Part model, mm, in its own coordinate system. A direction names the side the tool comes from. Give positions to 0.01 mm unless a question says otherwise; leave off trailing zeros. Order: outer loops, then holes, each group sorted by start corner. A loop starts at its lowest first (then second) coordinate and runs counter-clockwise, first axis right, second up. Notation, with made-up numbers: (5, -20) -> (40, -20) arc R25 ccw to (40, 13) -> close; hole circle Ø6 at (24.5, 42.25). An arc over 180 degrees is marked (long way). Write item = value, one per line. Start each with the question number.
(1) Saw through at B-B, the plane x = -22. List the corners of the cut face in (y, z), then the cut area to 3 significant figures.
(2) Flat gauge pins, fed straight in: pin 1 (1.3 mm diameter, centred on x = -43.5, z = 29, fed in from -Y); pin 2 (1 mm diameter, centred on x = -1, z = -31, fed in from -Y); pin 3 (1.8 mm diameter, centred on x = -45.83, z = -30.48, fed in from +Y); pin 4 (1.6 mm diameter, centred on y = 2, z = 3, fed in from +X). Where does each tip first touch, or does it go through?
(3) Two-plate mould, pull along X, no slides. Class faces 4 (the flat face through (1, -2, -29.813)), 5 (the flat face through (-41.632, 2, -31)), 6 (the cylindrical face through (43.43, -0.161, -28.686)), 7 (the flat face through (42.77, -1, 0)): pulls with the +X half, pulls with the -X half, needs draft (parallel to the pull), parting line crosses it, or undercut.
(4) Saw through at A-A, the plane z = -6. List the corners of the cut face in (x, y).
(5) Which spindle directions (+Z, -Z, +X, -X, +Y, -Y) get a long thin tool onto all of the face, cutting with end or side? Do faces 1 (the cylindrical face through (-43.454, -0.161, -28.654)), 2 (the cylindrical face through (45.09, 0.49, -26.23)), 3 (the cylindrical face through (-43.473, -2.058, 28.63)). Say none if no direction does.
(6) Probe line 1 along X through (y, z) = (-0.45, 21.5); line 2 along Z through (x, y) = (-11.5, -0.15); line 3 along X through (y, z) = (-2.2, -30.48). List the from-to ranges inside material, lowest first. Write a range as from..to.
from build123d import *

# Parameters (mm, degrees)
SKETCH1_W             = 83.263532188
SKETCH1_H             = 2
BOSS_EXTRUDE1_DEPTH   = 2.4732
BOSS_EXTRUDE1_2_DEPTH = 2.4732
SKETCH1_3_W           = 85.5392
SKETCH1_3_H           = 56.126
BOSS_EXTRUDE2_DEPTH   = 1
BOSS_EXTRUDE3_START   = -3.29023885
SKETCH1_4_W           = 85.5392
SKETCH1_4_H           = 56.126
BOSS_EXTRUDE3_DEPTH   = 3.29023885
BOSS_EXTRUDE4_START   = -3.290239
BOSS_EXTRUDE4_DEPTH   = 2
FILLET1_R             = 2
FILLET2_R             = 2
SKETCH2_R             = 3
CUT_EXTRUDE1_DEPTH    = 3
CUT_EXTRUDE2_START    = -2
SKETCH2_3_R           = 3
CUT_EXTRUDE2_DEPTH    = 2.5


with BuildPart() as part:
    # Sketch1 → Boss-Extrude1 (new body)
    with BuildSketch(Plane(origin=(0, 0, 0), x_dir=(1, 0, 0), z_dir=(0, 1, 0))):
        with Locations((0, 30.813)):
            Rectangle(SKETCH1_W, SKETCH1_H)
    extrude(amount=BOSS_EXTRUDE1_DEPTH)



with BuildPart() as body_2:
    # Sketch1 → Boss-Extrude1 2 (new body)
    with BuildSketch(Plane(origin=(0, 0, 0), x_dir=(1, 0, 0), z_dir=(0, 1, 0))):
        Polygon((-44.5196, -29.813), (-44.5196, 25.629766094), (-46.5196, 25.629766094), (-46.5196, -31.813), (46.5196, -31.813), (46.5196, 25.629766094), (44.5196, 25.629766094), (44.5196, -29.813), align=None)
    extrude(amount=BOSS_EXTRUDE1_2_DEPTH)


with BuildPart() as part_1:
    add(part.part)

    add(body_2.part)  # Boss-Extrude2 merges body 2
    # Sketch1<3> → Boss-Extrude2 (add)
    with BuildSketch(Plane(origin=(0, 0, 0), x_dir=(1, 0, 0), z_dir=(0, 1, 0))):
        with BuildLine():
            Line((41.631766094, 29.813), (-41.631766094, 29.813))
            Line((-41.631766094, 29.813), (-43.424920204, 29.813))
            ThreePointArc((-43.424920204, 29.813), (-43.834386894, 28.979884149), (-44.5196, 28.353603069))
            Line((-44.5196, 28.353603069), (-44.5196, 25.629766094))
            Line((-44.5196, 25.629766094), (-44.5196, -29.813))
            Line((-44.5196, -29.813), (44.5196, -29.813))
            Line((44.5196, -29.813), (44.5196, 25.629766094))
            Line((44.5196, 25.629766094), (44.5196, 28.353603069))
            ThreePointArc((44.5196, 28.353603069), (43.834386894, 28.979884149), (43.424920204, 29.813))
            Line((43.424920204, 29.813), (41.631766094, 29.813))
        make_face()
        Rectangle(SKETCH1_3_W, SKETCH1_3_H, mode=Mode.SUBTRACT)
    extrude(amount=BOSS_EXTRUDE2_DEPTH)

    # Sketch1<4> → Boss-Extrude3 (add)
    with BuildSketch(Plane(origin=(0, 0, 0), x_dir=(1, 0, 0), z_dir=(0, 1, 0)).offset(BOSS_EXTRUDE3_START)):
        with BuildLine():
            Line((41.631766094, 29.813), (-41.631766094, 29.813))
            Line((-41.631766094, 29.813), (-43.424920204, 29.813))
            ThreePointArc((-43.424920204, 29.813), (-43.834386894, 28.979884149), (-44.5196, 28.353603069))
            Line((-44.5196, 28.353603069), (-44.5196, 25.629766094))
            Line((-44.5196, 25.629766094), (-44.5196, -29.813))
            Line((-44.5196, -29.813), (44.5196, -29.813))
            Line((44.5196, -29.813), (44.5196, 25.629766094))
            Line((44.5196, 25.629766094), (44.5196, 28.353603069))
            ThreePointArc((44.5196, 28.353603069), (43.834386894, 28.979884149), (43.424920204, 29.813))
            Line((43.424920204, 29.813), (41.631766094, 29.813))
        make_face()
        Rectangle(SKETCH1_4_W, SKETCH1_4_H, mode=Mode.SUBTRACT)
    extrude(amount=BOSS_EXTRUDE3_DEPTH)

    # Sketch1<5> → Boss-Extrude4 (add)
    with BuildSketch(Plane(origin=(0, 0, 0), x_dir=(1, 0, 0), z_dir=(0, 1, 0)).offset(BOSS_EXTRUDE4_START)):
        with BuildLine():
            ThreePointArc((-43.3343, 30.48), (-43.524601169, 31.436708581), (-44.066533047, 32.247766953))
            ThreePointArc((-44.066533047, 32.247766953), (-47.602066953, 32.247766953), (-47.602066953, 28.712233047))
            ThreePointArc((-47.602066953, 28.712233047), (-46.123213969, 27.996750371), (-44.5196, 28.353603069))
            Line((-44.5196, 28.353603069), (-44.5196, 29.757806183))
            ThreePointArc((-44.5196, 29.757806183), (-47.287236681, 30.852793509), (-44.3343, 30.48))
            ThreePointArc((-44.3343, 30.48), (-44.373937666, 30.137448026), (-44.490755806, 29.813))
            Line((-44.490755806, 29.813), (-43.424920204, 29.813))
            ThreePointArc((-43.424920204, 29.813), (-43.357058642, 30.143436105), (-43.3343, 30.48))
        make_face()
        with BuildLine():
            ThreePointArc((-44.5196, 28.353603069), (-43.834386894, 28.979884149), (-43.424920204, 29.813))
            Line((-43.424920204, 29.813), (-44.490755806, 29.813))
            ThreePointArc((-44.490755806, 29.813), (-44.504891433, 29.785253383), (-44.5196, 29.757806183))
            Line((-44.5196, 29.757806183), (-44.5196, 28.353603069))
        make_face()
        with BuildLine():
            ThreePointArc((-44.5196, 28.353603069), (-46.123213969, 27.996750371), (-47.602066953, 28.712233047))
            Line((-47.602066953, 28.712233047), (-44.5196, 25.629766094))
            Line((-44.5196, 25.629766094), (-44.5196, 28.353603069))
        make_face()
        with BuildLine():
            Line((-41.631766094, 29.813), (-44.066533047, 32.247766953))
            ThreePointArc((-44.066533047, 32.247766953), (-43.524601169, 31.436708581), (-43.3343, 30.48))
            ThreePointArc((-43.3343, 30.48), (-43.357058642, 30.143436105), (-43.424920204, 29.813))
            Line((-43.424920204, 29.813), (-41.631766094, 29.813))
        make_face()
        with BuildLine():
            ThreePointArc((44.066533047, 32.247766953), (43.416829986, 31.117054732), (43.424920204, 29.813))
            Line((43.424920204, 29.813), (44.490755806, 29.813))
            ThreePointArc((44.490755806, 29.813), (45.491748026, 31.940362334), (47.3343, 30.48))
            ThreePointArc((47.3343, 30.48), (46.207093509, 29.027063319), (44.5196, 29.757806183))
            Line((44.5196, 29.757806183), (44.5196, 28.353603069))
            ThreePointArc((44.5196, 28.353603069), (46.123213969, 27.996750371), (47.602066953, 28.712233047))
            ThreePointArc((47.602066953, 28.712233047), (48.143998831, 29.523291419), (48.3343, 30.48))
            ThreePointArc((48.3343, 30.48), (46.791008581, 32.789698831), (44.066533047, 32.247766953))
        make_face()
        with BuildLine():
            Line((44.490755806, 29.813), (43.424920204, 29.813))
            ThreePointArc((43.424920204, 29.813), (43.834386894, 28.979884149), (44.5196, 28.353603069))
            Line((44.5196, 28.353603069), (44.5196, 29.757806183))
            ThreePointArc((44.5196, 29.757806183), (44.504891433, 29.785253383), (44.490755806, 29.813))
        make_face()
        with BuildLine():
            Line((44.066533047, 32.247766953), (41.631766094, 29.813))
            Line((41.631766094, 29.813), (43.424920204, 29.813))
            ThreePointArc((43.424920204, 29.813), (43.416829986, 31.117054732), (44.066533047, 32.247766953))
        make_face()
        with BuildLine():
            ThreePointArc((47.602066953, 28.712233047), (46.123213969, 27.996750371), (44.5196, 28.353603069))
            Line((44.5196, 28.353603069), (44.5196, 25.629766094))
            Line((44.5196, 25.629766094), (47.602066953, 28.712233047))
        make_face()
    extrude(amount=BOSS_EXTRUDE4_DEPTH)

    # Fillet1
    # the kernel refuses this fillet: 2 mm, written as the material it adds along each edge
    with BuildSketch(Plane(origin=(44.5196, 0, -25.629766094), x_dir=(0, 0, -1), z_dir=(0, 1, 0))) as fillet1_piece_1:
        with BuildLine():
            CenterArc((FILLET1_R, -FILLET1_R), FILLET1_R, 90, 90)
            Line((0, -FILLET1_R), (0, 0))
            Line((0, 0), (FILLET1_R, 0))
        make_face()
    extrude(amount=1)
    with BuildSketch(Plane(origin=(41.631766094, 0, -29.813), x_dir=(0, 0, -1), z_dir=(0, 1, 0))) as fillet1_piece_2:
        with BuildLine():
            CenterArc((1.989274938, -2), FILLET1_R, 90, 84.063686733)
            Line((0, -1.79315411), (0, 0))
            Line((0, 0), (1.989274938, 0))
        make_face()
    extrude(amount=1)
    with BuildSketch(Plane(origin=(-41.631766094, 0, -29.813), x_dir=(-1, 0, 0), z_dir=(0, 1, 0))) as fillet1_piece_3:
        with BuildLine():
            CenterArc((2, -1.989274938), FILLET1_R, 95.936313267, 84.063686733)
            Line((0, -1.989274938), (0, 0))
            Line((0, 0), (1.79315411, 0))
        make_face()
    extrude(amount=1)
    with BuildSketch(Plane(origin=(-44.5196, 0, -25.629766094), x_dir=(0, 0, -1), z_dir=(0, 1, 0))) as fillet1_piece_4:
        with BuildLine():
            CenterArc((FILLET1_R, FILLET1_R), FILLET1_R, 180, 90)
            Line((0, FILLET1_R), (0, 0))
            Line((0, 0), (FILLET1_R, 0))
        make_face()
    extrude(amount=1)

    # Fillet2
    fillet2_edges = [part_1.edges().sort_by_distance(p)[0] for p in [
        (-44.5196, 1.7366, 29.813),
        (44.5196, 1.7366, 29.813),
    ]]
    fillet(fillet2_edges, radius=FILLET2_R)

    # Sketch2 → Cut-Extrude1 (cut)
    with BuildSketch(Plane(origin=(0, -1.29023885, 0), x_dir=(1, 0, 0), z_dir=(0, 1, 0))):
        with Locations((-45.8343, 30.48)):
            Circle(SKETCH2_R)
        with Locations((45.8343, 30.48)):
            Circle(SKETCH2_R)
    extrude(amount=CUT_EXTRUDE1_DEPTH, mode=Mode.SUBTRACT)

    # Sketch2<3> → Cut-Extrude2 (cut)
    with BuildSketch(Plane(origin=(0, -1.29023885, 0), x_dir=(1, 0, 0), z_dir=(0, 1, 0)).offset(CUT_EXTRUDE2_START)):
        with Locations((-45.8343, -30.48)):
            Circle(SKETCH2_3_R)
        with Locations((45.8343, -30.48)):
            Circle(SKETCH2_3_R)
    extrude(amount=CUT_EXTRUDE2_DEPTH, mode=Mode.SUBTRACT)


solid = part_1.part
Results list:
q1.outline = (-3.29, -29.81) -> (0, -29.81) -> (0, -31.81) -> (2.47, -31.81) -> (2.47, -29.81) -> (1, -29.81) -> (1, -28.06) -> (-3.29, -28.06) -> close; (-3.29, 28.06) -> (1, 28.06) -> (1, 29.81) -> (2.47, 29.81) -> (2.47, 31.81) -> (0, 31.81) -> (0, 29.81) -> (-3.29, 29.81) -> close
q1.area = 24.9 mm^2
q2.pin_1 = -3.29
q2.pin_2 = 0
q2.pin_3 = through
q2.pin_4 = 46.52
q3.face_4 = undercut
q3.face_5 = pulls with the -X half
q3.face_6 = pulls with the +X half
q3.face_7 = undercut
q4.outline = (-46.52, 0) -> (-44.52, 0) -> (-44.52, -3.29) -> (-42.77, -3.29) -> (-42.77, 1) -> (-44.52, 1) -> (-44.52, 2.47) -> (-46.52, 2.47) -> close; (42.77, -3.29) -> (44.52, -3.29) -> (44.52, 0) -> (46.52, 0) -> (46.52, 2.47) -> (44.52, 2.47) -> (44.52, 1) -> (42.77, 1) -> close
q5.face_1 = -Z, -X, +Y
q5.face_2 = -Z, +X, +Y
q5.face_3 = +Z, -X, -Y
q6.line_1 = -44.52..-42.77, 42.77..44.52
q6.line_2 = -29.81..-28.06, 28.06..29.81
q6.line_3 = -48.33..-47.33, -44.33..-42.3, 42.3..44.33, 47.33..48.33
